from build123d import *

# Parameters (mm, degrees)
F0_W     = 63.5
F0_H     = 63.5
F1_DEPTH = 96.012
F3_DEPTH = 73.914


with BuildPart() as f1:
    # F0 (on Front) → F1 (new body)
    with BuildSketch(Plane.XZ):
        Rectangle(F0_W, F0_H)
        Polygon((-15.875, 15.875), (15.875, 15.875), (15.875, 13.49375), (25.4, 13.49375), (25.4, -13.49375), (15.875, -13.49375), (15.875, -15.875), (-15.875, -15.875), (-15.875, -13.49375), (-25.4, -13.49375), (-25.4, 13.49375), (-15.875, 13.49375), align=None, mode=Mode.SUBTRACT)
    extrude(amount=F1_DEPTH)

    # F2 (on face) → F3 (cut)
    with BuildSketch(Plane.YZ.offset(31.75)):
        with BuildLine():
            ThreePointArc((-79.756, 6.35), (-86.106, 0), (-79.756, -6.35))
            Line((-79.756, -6.35), (-16.256, -6.35))
            ThreePointArc((-16.256, -6.35), (-9.906, 0), (-16.256, 6.35))
            Line((-16.256, 6.35), (-79.756, 6.35))
        make_face()
    extrude(amount=-F3_DEPTH, mode=Mode.SUBTRACT)


solid = f1.part
Model file for the job. Use its own axes, mm. A direction names the side the tool comes from. Coordinates: 2 decimals unless noted, no trailing zeros. Loops run counter-clockwise (first coordinate to the right, second up) from the corner with the lowest first, then second, coordinate; pieces in that order, holes last. Notation, with made-up numbers: (39.25, 71.25) -> (52.25, 71.25) arc R23 cw to (52.25, 89.25) -> close; hole circle Ø2 at (85, 75.5). An arc over 180 degrees is marked (long way). Use one line per item in the form item = value. Start each with the question number.
(1) Flat gauge pins, fed straight in: pin 1 (6 mm diameter, centred on y = -12, z = -3, fed in from +X); pin 2 (1.5 mm diameter, centred on x = -14.5, z = -15, fed in from +Y). Where does each tip first touch, or does it go through?
(2) Cut at B-B on z = 0. Give the cut face in (x, y).
(3) Cut at A-A on y = -66. Give the cut face in (x, z) (3 decimals), and give its area (3 significant figures).
(4) Cut at D-D on y = -85. Give the cut face in (x, z) (3 decimals).
(5) Tool access for faces 1 (the cylindrical face through (-28.531, -86.104, 0.14)), 2 (the flat face through (-15.875, -47, -15)), 3 (the flat face through (0, 0, 22)): list every direction of +Z, -Z, +X, -X, +Y, -Y with a clear straight run to the whole face (end or side of a thin tool).
(6) Probe probe 1 along Z at (x, y) = (-17, -12.5); probe 2 along Z at (x, y) = (-14.5, -7.5) (3 decimals); probe 3 along X at (y, z) = (-72, -8.5). List the from-to ranges inside material, lowest first. Write a range as from..to.
(7) Pull direction Z, two halves, no side cores. Call faces 4 (the flat face through (0, -96.012, 22)), 5 (the flat face through (-21, -47, 13.494)): pulls with the +Z half, pulls with the -Z half, needs draft (parallel to the pull), parting line crosses it, or undercut.
(8) Cut at C-C on x = 11. Give the cut face in (y, z) (3 decimals).
Values:
q1.pin_1 = 31.75
q1.pin_2 = through
q2.outline = (-31.75, -96.01) -> (-25.4, -96.01) -> (-25.4, -86.11) -> (-31.75, -86.11) -> close; (-31.75, -9.91) -> (-25.4, -9.91) -> (-25.4, 0) -> (-31.75, 0) -> close; (25.4, -96.01) -> (31.75, -96.01) -> (31.75, -86.11) -> (25.4, -86.11) -> close; (25.4, -9.91) -> (31.75, -9.91) -> (31.75, 0) -> (25.4, 0) -> close
q3.outline = (-31.75, -31.75) -> (31.75, -31.75) -> (31.75, -6.35) -> (25.4, -6.35) -> (25.4, -13.494) -> (15.875, -13.494) -> (15.875, -15.875) -> (-15.875, -15.875) -> (-15.875, -13.494) -> (-25.4, -13.494) -> (-25.4, -6.35) -> (-31.75, -6.35) -> close; (-31.75, 6.35) -> (-25.4, 6.35) -> (-25.4, 13.494) -> (-15.875, 13.494) -> (-15.875, 15.875) -> (15.875, 15.875) -> (15.875, 13.494) -> (25.4, 13.494) -> (25.4, 6.35) -> (31.75, 6.35) -> (31.75, 31.75) -> (-31.75, 31.75) -> close
q3.area = 2,350 mm2
q4.outline = (-31.75, -31.75) -> (31.75, -31.75) -> (31.75, -3.581) -> (25.4, -3.581) -> (25.4, -13.494) -> (15.875, -13.494) -> (15.875, -15.875) -> (-15.875, -15.875) -> (-15.875, -13.494) -> (-25.4, -13.494) -> (-25.4, -3.581) -> (-31.75, -3.581) -> close; (-31.75, 3.581) -> (-25.4, 3.581) -> (-25.4, 13.494) -> (-15.875, 13.494) -> (-15.875, 15.875) -> (15.875, 15.875) -> (15.875, 13.494) -> (25.4, 13.494) -> (25.4, 3.581) -> (31.75, 3.581) -> (31.75, 31.75) -> (-31.75, 31.75) -> close
q5.face_1 = +X, -X
q5.face_2 = +Y, -Y
q5.face_3 = +Z, -Z, +X, -X, +Y
q6.probe_1 = -31.75..-13.49, 13.49..31.75
q6.probe_2 = -31.75..-15.875, 15.875..31.75
q6.probe_3 = -31.75..-25.4, 25.4..31.75
q7.face_4 = needs draft
q7.face_5 = undercut
q8.outline = (-96.012, -31.75) -> (0, -31.75) -> (0, -15.875) -> (-96.012, -15.875) -> close; (-96.012, 15.875) -> (0, 15.875) -> (0, 31.75) -> (-96.012, 31.75) -> close
